Here's how the part is built. I have some questions about the finished solid (model axes, mm). Face numbers are marked on the shaded views. A direction names the side the tool comes from. Coordinates: 2 decimals unless noted, no trailing zeros. Write each loop counter-clockwise with the first axis right and the second up, starting at its lowest first coordinate (ties: lowest second). Pieces come first, ordered by that corner, then holes. Notation, with made-up numbers: (1.25, 3) - (29.25, 3) arc R22 ccw to (29.25, 22) - close; hole circle Ø5 at (-33, -1). An arc over 180 degrees is marked (long way). Answer in a Markdown table with one row per item. Add a question column.
Item 1: Imagine slicing it at D-D (x = 7). Please give me the cut outline in (y, z).
Item 2: Which directions (+Z, -Z, +X, -X, +Y, -Y) give clear straight access to the entire face, cutting with the end or side of a thin tool? Please do the marked faces 4, 5 and 6.
Item 3: If I drill on probe 1 along Z at (x, y) = (13.5, 16); probe 2 along X at (y, z) = (4, -16); probe 3 along X at (y, z) = (21.5, -12.25), over which ranges is the centre line in solid material (lowest first)? Write a range as from..to.
Item 4: I'm going to push flat-ended pins straight in: pin 1 (3.5 mm diameter, centred on x = 10, y = 8.5, fed in from -Z); pin 2 (9 mm diameter, centred on y = 3, z = -12.5, fed in from -X); pin 3 (11.5 mm diameter, centred on y = 18, z = -5, fed in from +X); pin 4 (8 mm diameter, centred on x = 8, z = -9, fed in from +Y). Where does each tip first touch, or does it pass through?
Item 5: Imagine slicing it at B-B (z = -14.75). Please give me the cut outline in (x, y), plus the area to 3 significant figures.
Item 6: We'd pull the mould along Z, two halves only. Please class the marked faces 1, 2 and 3: +Z half, -Z half, draft (parallel to the pull), parting line (faces both ways), or undercut.
Item 7: Imagine slicing it at C-C (y = 15). Please give me the cut outline in (x, z), plus the area to 3 significant figures.
Item 8: Imagine slicing it at A-A (x = 13.5). Please give me the cut outline in (y, z), plus the area to 3 significant figures.
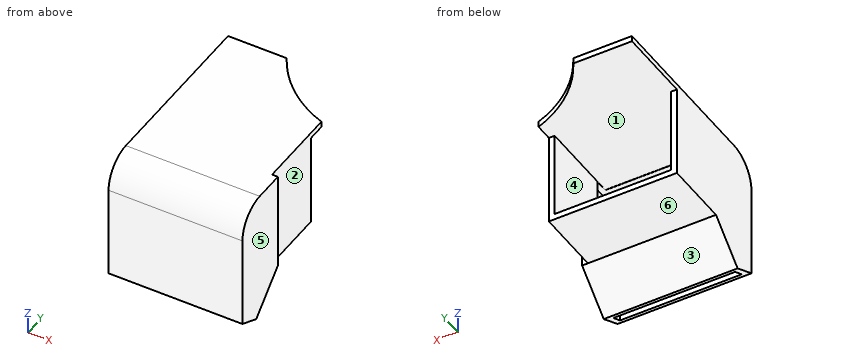
from build123d import *

# Parameters (mm, degrees)
SKETCH1_W           = 23
SKETCH1_H           = 17
BOSS_EXTRUDE1_DEPTH = 10.256
BOSS_EXTRUDE2_DEPTH = 23
SHELL1_T            = -1.044
SKETCH3_W           = 22
SKETCH3_H           = 17
BOSS_EXTRUDE3_DEPTH = 24.294
SHELL2_START        = 1
SHELL2_OUTLINE_W    = 24.338
SHELL2_OUTLINE_H    = 15
SHELL2_DEPTH        = 20
SKETCH4_W           = 20
SKETCH4_H           = 15
CUT_EXTRUDE1_DEPTH  = 3.294
SKETCH5_W           = 16
SKETCH5_H           = 13
CUT_EXTRUDE2_DEPTH  = 26.294
CUT_EXTRUDE3_DEPTH  = 26.294
FILLET1_R           = 5
FILLET2_R           = 5


# Read off the part's stored shape, not the designer's step: Shell2
with BuildPart() as part:
    # Sketch1 → Boss-Extrude1 (new body)
    with BuildSketch(Plane(origin=(0, 0, 0), x_dir=(1, 0, 0), z_dir=(0, 1, 0))):
        with Locations((11.5, 8.5)):
            Rectangle(SKETCH1_W, SKETCH1_H)
    extrude(amount=BOSS_EXTRUDE1_DEPTH)

    # Sketch2 → Boss-Extrude2 (add)
    with BuildSketch(Plane(origin=(23, 0, 0), x_dir=(0, 0, -1), z_dir=(1, 0, 0))):
        Polygon((17, 0), (20.918, 0), (22.816626616, 4.000300111), (17, 10.256), align=None)
    extrude(amount=-BOSS_EXTRUDE2_DEPTH)

    # Shell1
    shell1_openings = [part.faces().sort_by_distance(p)[0] for p in [
        (11.5, 2.000150055, -21.867313308),
    ]]
    offset(amount=SHELL1_T, openings=shell1_openings, kind=Kind.INTERSECTION)

    # Sketch3 → Boss-Extrude3 (add)
    with BuildSketch(Plane(origin=(0, 10.256, 0), x_dir=(1, 0, 0), z_dir=(0, 1, 0))):
        with Locations((11, 8.5)):
            Rectangle(SKETCH3_W, SKETCH3_H)
    extrude(amount=BOSS_EXTRUDE3_DEPTH)

    # Shell2 outline → Shell2 (cut)
    with BuildSketch(Plane.YZ.offset(SHELL2_START)):
        with Locations((22.381, -8.5)):
            Rectangle(SHELL2_OUTLINE_W, SHELL2_OUTLINE_H)
    extrude(amount=SHELL2_DEPTH, mode=Mode.SUBTRACT)

    # Sketch4 → Cut-Extrude1 (cut)
    with BuildSketch(Plane(origin=(0, 10.212, 0), x_dir=(1, 0, 0), z_dir=(0, 1, 0))):
        with Locations((11, 8.5)):
            Rectangle(SKETCH4_W, SKETCH4_H)
    extrude(amount=-CUT_EXTRUDE1_DEPTH, mode=Mode.SUBTRACT)

    # Sketch5 → Cut-Extrude2 (cut)
    with BuildSketch(Plane(origin=(22, 0, 0), x_dir=(0, 0, -1), z_dir=(1, 0, 0))):
        with Locations((9, 28.05)):
            Rectangle(SKETCH5_W, SKETCH5_H)
    extrude(amount=-CUT_EXTRUDE2_DEPTH, mode=Mode.SUBTRACT)

    # Sketch6 → Cut-Extrude3 (cut)
    with BuildSketch(Plane.XY):
        with BuildLine():
            Line((22, 34.55), (10.070124752, 34.55))
            ThreePointArc((10.070124752, 34.55), (15.112523328, 28.440572535), (22, 24.5273191))
            Line((22, 24.5273191), (22, 34.55))
        make_face()
    extrude(amount=-CUT_EXTRUDE3_DEPTH, mode=Mode.SUBTRACT)

    # Fillet1
    fillet1_edges = [part.edges().sort_by_distance(p)[0] for p in [
        (11.5, 0, 0),
    ]]
    fillet(fillet1_edges, radius=FILLET1_R)

    # Fillet2
    fillet2_edges = [part.edges().sort_by_distance(p)[0] for p in [
        (11.5, 1.044, -1.044),
    ]]
    fillet(fillet2_edges, radius=FILLET2_R)


solid = part.part
Here are the results:
| question | item | result |
|---|---|---|
| 1 | outline | (0, -20.92) - (1.04, -21.41) - (1.04, -6.04) arc R5 cw to (6.04, -1.04) - (6.92, -1.04) - (6.92, -1) - (34.55, -1) - (34.55, 0) - (5, 0) arc R5 ccw to (0, -5) - close; (2.99, -22.33) - (4, -22.82) - (10.26, -17) - (21.55, -17) - (21.55, -16) - (9.21, -16) - (9.21, -16.55) - close |
| 2 | face 4 | +Y |
| 2 | face 5 | +Z, -Z, +X, +Y, -Y |
| 2 | face 6 | -Z, +X, -X, +Y |
| 3 | probe 1 | z = -17..-16, -1..0 |
| 3 | probe 2 | x = 0..1.04, 21.96..23 |
| 3 | probe 3 | x = 0..1, 21..22 |
| 4 | pin 1 | stops at z = -20.26 |
| 4 | pin 2 | stops at x = 0 |
| 4 | pin 3 | stops at x = 22 |
| 4 | pin 4 | stops at y = 1.15 |
| 5 | outline | (0, 0) - (23, 0) - (23, 10.26) - (22, 10.26) - (22, 21.55) - (21, 21.55) - (21, 9.21) - (21.96, 9.21) - (21.96, 1.04) - (1.04, 1.04) - (1.04, 6.92) - (1, 6.92) - (1, 21.55) - (0, 21.55) - close |
| 5 | area | 66.7 mm2 |
| 6 | face 1 | undercut |
| 6 | face 2 | draft |
| 6 | face 3 | -Z half |
| 7 | outline | (0, -17) - (22, -17) - (22, 0) - (0, 0) - close; hole (1, -16) - (21, -16) - (21, -1) - (1, -1) - close |
| 7 | area | 74.0 mm2 |
| 8 | outline | (0, -20.92) - (1.04, -21.41) - (1.04, -6.04) arc R5 cw to (6.04, -1.04) - (6.92, -1.04) - (6.92, -1) - (29.94, -1) - (29.94, 0) - (5, 0) arc R5 ccw to (0, -5) - close; (2.99, -22.33) - (4, -22.82) - (10.26, -17) - (21.55, -17) - (21.55, -16) - (9.21, -16) - (9.21, -16.55) - close |
| 8 | area | 72.2 mm2 |
